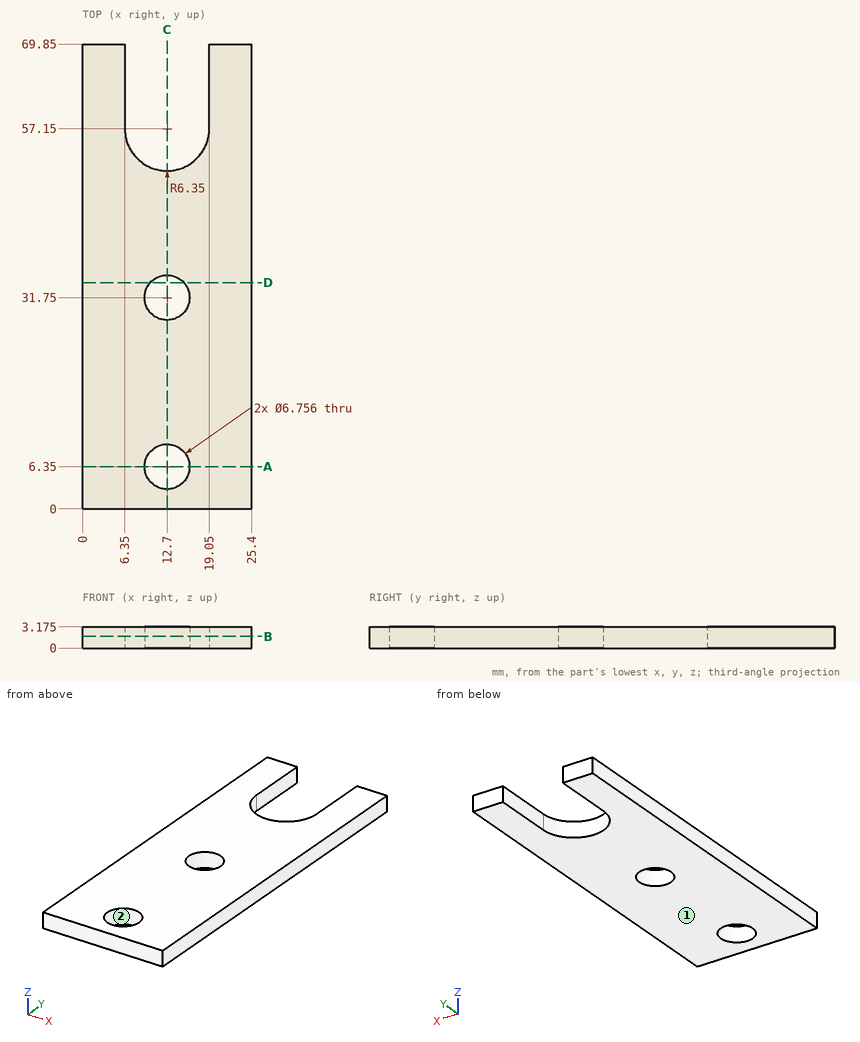
For this review, use the dimensioned drawing (mm, ordinates from the lowest corner) and the shaded views. Round coordinates to 2 decimals unless told otherwise and drop trailing zeros. Write each loop counter-clockwise with the first axis right and the second up, starting at its lowest first coordinate (ties: lowest second). Pieces come first, ordered by that corner, then holes. Notation, with made-up numbers: (-3, 34) - (50, 34) arc R6 ccw to (50, 41) - close; hole circle Ø2 at (47.5, -8.75). An arc over 180 degrees is marked (long way). One line per item, written item: value. Start each with the question number.
1. To check wall thickness, follow L1, parallel to Y at x = 12.7, z = 2; L2, parallel to Y at x = 14.75, z = 0.2 (1 decimal); L3, parallel to X at y = 64, z = 1.3. State the ranges of each line that lie inside material, in increasing order. Write a range as from..to.
2. Clearance check with a flat-ended pin moving along its axis: P1, Ø3, axis at x = 10, y = 53.5, coming from the -Z side. State where the tip first meets the part, or that it passes through.
3. Consider section B-B on z = 1.75. Write out the cut boundary in (x, y), and give its area (3 significant figures).
4. Consider section C-C on x = 12.7. Write out the cut boundary in (y, z) (1 decimal), and give its area (3 significant figures).
5. Consider section A-A on y = 6.35. Write out the cut boundary in (x, z) (1 decimal), and give its area (3 significant figures).
6. The part is to be moulded in two halves that separate along X. For the marked faces 1 and 2, say which applies: released by +X, released by -X, zero draft, split by the parting line, or undercut.
7. Consider section D-D on y = 34. Write out the cut boundary in (x, z) (1 decimal).
Checks:
1. L1: y = 0..2.97, 9.73..28.37, 35.13..50.8
1. L2: y = 0..3.7, 9..29.1, 34.4..51.1
1. L3: x = 0..6.35, 19.05..25.4
2. P1: passes through
3. outline: (0, 0) - (25.4, 0) - (25.4, 69.85) - (19.05, 69.85) - (19.05, 57.15) arc R6.35 cw to (6.35, 57.15) - (6.35, 69.85) - (0, 69.85) - close; hole circle Ø6.76 at (12.7, 6.35); hole circle Ø6.76 at (12.7, 31.75)
3. area: 1,480 mm^2
4. outline: (0, 0) - (3, 0) - (3, 3.2) - (0, 3.2) - close; (9.7, 0) - (28.4, 0) - (28.4, 3.2) - (9.7, 3.2) - close; (35.1, 0) - (50.8, 0) - (50.8, 3.2) - (35.1, 3.2) - close
4. area: 118 mm^2
5. outline: (0, 0) - (9.3, 0) - (9.3, 3.2) - (0, 3.2) - close; (16.1, 0) - (25.4, 0) - (25.4, 3.2) - (16.1, 3.2) - close
5. area: 59.2 mm^2
6. face 1: zero draft
6. face 2: undercut
7. outline: (0, 0) - (10.2, 0) - (10.2, 3.2) - (0, 3.2) - close; (15.2, 0) - (25.4, 0) - (25.4, 3.2) - (15.2, 3.2) - close
